from build123d import *

# Parameters (mm, degrees)
SKETCH_1_W                     = 18
SKETCH_1_H                     = 37
EXTRUDE_1_DEPTH                = 65.5
SKETCH_2_R                     = 5
CUT_EXTRUDE_1_DEPTH            = 0.5
CUT_EXTRUDE_START              = -0.5
SKETCH_3_R                     = 5
CUT_EXTRUDE_2_DEPTH            = 0.5
SKETCH_4_R                     = 1.5
CUT_EXTRUDE_3_DEPTH            = 78.351470574
SKETCH_5_W                     = 1.835428096
SKETCH_5_H                     = 2.75652024
CUT_EXTRUDE_4_DEPTH            = 78.351470574
SKETCH_6_W                     = 5
SKETCH_6_H                     = 17
CUT_EXTRUDE_5_DEPTH            = 78.351470574
SKETCH_7_W                     = 8
SKETCH_7_H                     = 12
CUT_EXTRUDE_6_DEPTH            = 78.351470574
SKETCH_8_R                     = 2.5
EXTRUDE_2_DEPTH                = 1.5
SKETCH_9_W                     = 17.5
SKETCH_9_H                     = 35.5
EXTRUDE_3_DEPTH                = 4.5
SKETCH_10_W                    = 7
SKETCH_10_H                    = 11
EXTRUDE_4_DEPTH                = 64
CUT_EXTRUDE_7_REACH            = 84.061
SKETCH_11_W                    = 4.5
SKETCH_11_H                    = 18.5
HOLE_WIZARD_M3_1_D             = 2.5
HOLE_WIZARD_M3_1_DEPTH         = 7.5
HOLE_WIZARD_M3_1_TIP           = 0.751075774
HOLE_WIZARD_M3_1_2_D           = 3.4
HOLE_WIZARD_M3_1_2_DEPTH       = 5
HOLE_WIZARD_M3_1_2_CBORE_D     = 6.5
HOLE_WIZARD_M3_1_2_CBORE_DEPTH = 3
CUT_EXTRUDE_8_REACH            = 84.172
SKETCH_16_R                    = 3
HOLE_WIZARD_M3_2_D             = 2.5
HOLE_WIZARD_M3_2_DEPTH         = 7.5
HOLE_WIZARD_M3_2_TIP           = 0.751075774


with BuildPart() as part:
    # 草图1 → 凸台-拉伸1 (new body)
    with BuildSketch(Plane(origin=(0, 0, 0), x_dir=(0, 0, -1), z_dir=(1, 0, 0))):
        with Locations((9, 18.5)):
            Rectangle(SKETCH_1_W, SKETCH_1_H)
    extrude(amount=EXTRUDE_1_DEPTH)

    # 草图2 → 切除-拉伸1 (cut)
    with BuildSketch(Plane.ZY):
        with Locations((-9, 11)):
            Circle(SKETCH_2_R)
    extrude(amount=-CUT_EXTRUDE_1_DEPTH, mode=Mode.SUBTRACT)

    # 草图3 → 切除-拉伸2 (cut)
    with BuildSketch(Plane(origin=(65.5, 0, 0), x_dir=(0, 0, -1), z_dir=(1, 0, 0)).offset(CUT_EXTRUDE_START)):
        with Locations(Location((9, 11, 0), (0, 0, 180))):
            Circle(SKETCH_3_R)
    extrude(amount=CUT_EXTRUDE_2_DEPTH, mode=Mode.SUBTRACT)

    # 草图4 → 切除-拉伸3 (cut, through all)
    with BuildSketch(Plane.ZY):
        with Locations((-13, 3)):
            Circle(SKETCH_4_R)
        with Locations(Location((-5, 3, 0), (0, 0, 180))):
            Circle(SKETCH_4_R)
    extrude(amount=-CUT_EXTRUDE_3_DEPTH, mode=Mode.SUBTRACT)

    # 草图5 → 切除-拉伸4 (cut, through all)
    with BuildSketch(Plane.ZY):
        with Locations((-13, 1.37826012)):
            Rectangle(SKETCH_5_W, SKETCH_5_H)
        with Locations((-5, 1.37826012)):
            Rectangle(SKETCH_5_W, SKETCH_5_H)
    extrude(amount=-CUT_EXTRUDE_4_DEPTH, mode=Mode.SUBTRACT)

    # 草图6 → 切除-拉伸5 (cut, through all)
    with BuildSketch(Plane.ZY):
        with Locations((-2.5, 28.5)):
            Rectangle(SKETCH_6_W, SKETCH_6_H)
    extrude(amount=-CUT_EXTRUDE_5_DEPTH, mode=Mode.SUBTRACT)

    # 草图7 → 切除-拉伸6 (cut, through all)
    with BuildSketch(Plane.ZY):
        with Locations((-9, 28)):
            Rectangle(SKETCH_7_W, SKETCH_7_H)
    extrude(amount=-CUT_EXTRUDE_6_DEPTH, mode=Mode.SUBTRACT)

    # 草图8 → 凸台-拉伸2 (add)
    with BuildSketch(Plane(origin=(65, 0, 0), x_dir=(0, 0, -1), z_dir=(1, 0, 0))):
        with Locations((9, 11)):
            Circle(SKETCH_8_R)
    extrude(amount=EXTRUDE_2_DEPTH)

    # 草图9 → 凸台-拉伸3 (add)
    with BuildSketch(Plane(origin=(66.5, 0, 0), x_dir=(0, 0, -1), z_dir=(1, 0, 0))):
        with Locations((8.25, 18.75)):
            Rectangle(SKETCH_9_W, SKETCH_9_H)
    extrude(amount=EXTRUDE_3_DEPTH)

    # 草图10 → 凸台-拉伸4 (add)
    with BuildSketch(Plane.ZY.offset(-66.5)):
        with Locations((-3, 28)):
            Rectangle(SKETCH_10_W, SKETCH_10_H)
    extrude(amount=EXTRUDE_4_DEPTH)

    # 草图11 → 切除-拉伸7 (cut, up to next)
    with BuildSketch(Plane(origin=(71, 0, 0), x_dir=(0, 0, -1), z_dir=(1, 0, 0)), mode=Mode.PRIVATE) as cut_extrude_7_sk1:
        with Locations((1.75, 10.25)):
            Rectangle(SKETCH_11_W, SKETCH_11_H)
    cut_extrude_7_tool1 = extrude(cut_extrude_7_sk1.sketch, amount=-CUT_EXTRUDE_7_REACH, mode=Mode.PRIVATE) & part.part
    add(cut_extrude_7_tool1.solids().sort_by_distance((71, 10.25, -1.75))[0], mode=Mode.SUBTRACT)

    # Hole Wizard M3 _1
    with Locations(Plane(origin=(71, 0, 0), x_dir=(0, 0, -1), z_dir=(1, 0, 0))):
        with Locations((13.5, 33), (3, 23)):
            Hole(HOLE_WIZARD_M3_1_D / 2, depth=HOLE_WIZARD_M3_1_DEPTH)
            with Locations((0, 0, -(HOLE_WIZARD_M3_1_DEPTH + HOLE_WIZARD_M3_1_TIP / 2))):  # 118° drill point
                Cone(0, HOLE_WIZARD_M3_1_D / 2, HOLE_WIZARD_M3_1_TIP, mode=Mode.SUBTRACT)

    # Hole Wizard M3 _1 2
    with Locations(Plane.XY.offset(-13)):
        with Locations((4, 28), (61.5, 28)):
            CounterBoreHole(HOLE_WIZARD_M3_1_2_D / 2, HOLE_WIZARD_M3_1_2_CBORE_D / 2, HOLE_WIZARD_M3_1_2_CBORE_DEPTH, depth=HOLE_WIZARD_M3_1_2_DEPTH)

    # 草图16 → 切除-拉伸8 (cut, up to next)
    with BuildSketch(Plane.XY.offset(0.5), mode=Mode.PRIVATE) as cut_extrude_8_sk1:
        with Locations((61, 28)):
            Circle(SKETCH_16_R)
    cut_extrude_8_tool1 = extrude(cut_extrude_8_sk1.sketch, amount=-CUT_EXTRUDE_8_REACH, mode=Mode.PRIVATE) & part.part
    add(cut_extrude_8_tool1.solids().sort_by_distance((61, 28, 0.5))[0], mode=Mode.SUBTRACT)

    # M3 螺纹孔2
    with Locations(Plane.XY.offset(0.5)):
        with Locations((28, 28), (48, 28)):
            Hole(HOLE_WIZARD_M3_2_D / 2, depth=HOLE_WIZARD_M3_2_DEPTH)
            with Locations((0, 0, -(HOLE_WIZARD_M3_2_DEPTH + HOLE_WIZARD_M3_2_TIP / 2))):  # 118° drill point
                Cone(0, HOLE_WIZARD_M3_2_D / 2, HOLE_WIZARD_M3_2_TIP, mode=Mode.SUBTRACT)


solid = part.part
Read the model definition and answer for the solid it produces. Units are mm, in the model's axes. A direction names the side the tool comes from. Give positions to 0.01 mm unless a question says otherwise; leave off trailing zeros. Write each loop counter-clockwise with the first axis right and the second up, starting at its lowest first coordinate (ties: lowest second). Pieces come first, ordered by that corner, then holes. Notation, with made-up numbers: (-40, -30) - (-2, -30) arc R15 cw to (-2, -11) - close; hole circle Ø4 at (-27, -25). An arc over 180 degrees is marked (long way). Use CSV: the item, a comma, the result in double quotes. Start each with the question number.
Item 1: The part is cut by section A-A, the plane x = 48. Give the vertices of the cut face in (y, z).
Item 2: For faces 1 (the flat face through (69, 10, -4)), 2 (the flat face through (32, 1, -12.082)), 3 (the flat face through (32, 20, -3)), 4 (the cylindrical face through (48.99, 27.24, -3.05)), 5 (the cylindrical face through (3.295, 24.827, -14.479)), determine the directions among +Z, -Z, +X, -X, +Y, -Y from which every point of the face is accessible in a straight line to the end or side of a thin tool.
Item 3: The mould has two halves that part along Z. Classify faces 6 (the flat face through (32, 18, -18)), 7 (the conical face through (62.88, 33.07, -13.71)), 8 (the flat face through (69, 1, -10)): pulls with the +Z half, pulls with the -Z half, needs draft (parallel to the pull), parting line crosses it, or undercut.
Item 4: Consider line 1 (Z direction, x = 40, y = 3); line 2 (Y direction, x = 61, z = -3); line 3 (X direction, y = 24, z = -15.5). Determine where each line is inside the solid, lowest interval first.
Item 5: Flat-ended cylindrical pins translate along their axes: P1, Ø6, axis at x = 54, z = -11.5, coming from the -Y side; P2, Ø3, axis at y = 10.5, z = -8, coming from the -X side; P3, Ø1.3, axis at x = 68, y = 7.5, coming from the +Z side; P4, Ø16, axis at x = 25.5, y = 11, coming from the +Z side. Find the tip coordinate at first contact, or state that the pin passes through.
Item 6: The part is cut by section B-B, the plane z = -9. Give the vertices of the cut face in (x, y), and give its area (3 significant figures).
Item 7: The part is cut by section D-D, the plane x = 21.5. Give the vertices of the cut face in (y, z).
Item 8: The part is cut by section C-C, the plane y = 11. Give the vertices of the cut face in (x, z).
Taken from the geometry:
1,outline,"(0, -18) - (37, -18) - (37, -5) - (34, -5) - (34, -13) - (22, -13) - (22, -5) - (20, -5) - (20, 0) - (0, 0) - (0, -4.08) - (1.81, -4.08) arc R1.5 cw (long way) to (1.81, -5.92) - (0, -5.92) - (0, -12.08) - (1.81, -12.08) arc R1.5 cw (long way) to (1.81, -13.92) - (0, -13.92) - close; (22.5, -6.5) - (26.75, -6.5) - (26.75, 0.5) - (22.5, 0.5) - close; (29.25, -6.5) - (33.5, -6.5) - (33.5, 0.5) - (29.25, 0.5) - close"
2,face 1,"+Z, +X, -Y"
2,face 2,"-X, -Y"
2,face 3,"+Z, -X"
2,face 4,"+Z"
2,face 5,"none"
3,face 6,"pulls with the -Z half"
3,face 7,"undercut"
3,face 8,"needs draft"
4,line 1,"-18 to -14.5, -11.5 to -6.5, -3.5 to 0"
4,line 2,"0 to 20, 22.5 to 25, 31 to 33.5"
4,line 3,"0 to 65.5, 66.5 to 71"
5,P1,"y = 0"
5,P2,"x = 0.5"
5,P3,"z = -4"
5,P4,"z = 0"
6,outline,"(0, 0) - (65.5, 0) - (65.5, 6) - (65, 6) - (65, 8.5) - (66.5, 8.5) - (66.5, 1) - (71, 1) - (71, 36.5) - (66.5, 36.5) - (66.5, 13.5) - (65, 13.5) - (65, 16) - (65.5, 16) - (65.5, 22) - (0, 22) - (0, 16) - (0.5, 16) - (0.5, 6) - (0, 6) - close; (0, 34) - (65.5, 34) - (65.5, 37) - (0, 37) - close"
6,area,"1,790 mm2"
7,outline,"(0, -18) - (37, -18) - (37, -5) - (34, -5) - (34, -13) - (22, -13) - (22, -5) - (20, -5) - (20, 0) - (0, 0) - (0, -4.08) - (1.81, -4.08) arc R1.5 cw (long way) to (1.81, -5.92) - (0, -5.92) - (0, -12.08) - (1.81, -12.08) arc R1.5 cw (long way) to (1.81, -13.92) - (0, -13.92) - close; (22.5, -6.5) - (33.5, -6.5) - (33.5, 0.5) - (22.5, 0.5) - close"
8,outline,"(0, -18) - (65.5, -18) - (65.5, -14) - (65, -14) - (65, -11.5) - (66.5, -11.5) - (66.5, -17) - (71, -17) - (71, -4) - (66.5, -4) - (66.5, -6.5) - (65, -6.5) - (65, -4) - (65.5, -4) - (65.5, 0) - (0, 0) - (0, -4) - (0.5, -4) - (0.5, -14) - (0, -14) - close"
